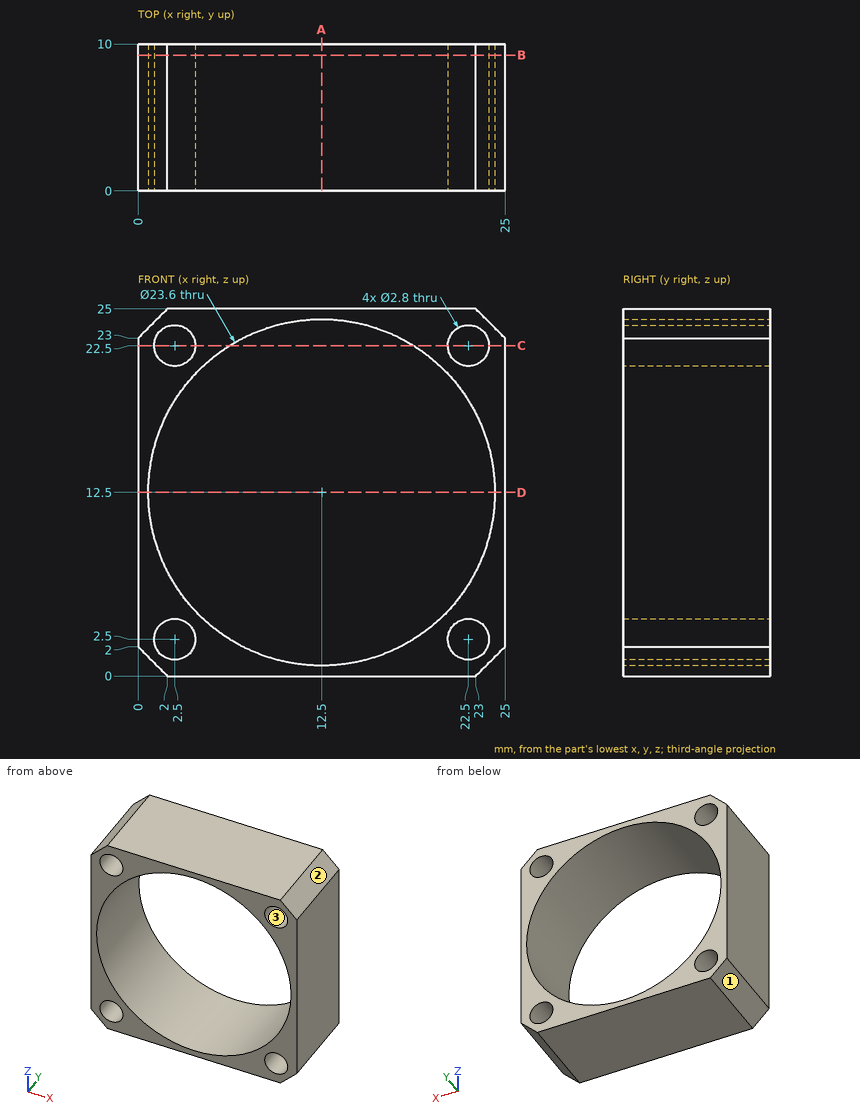
Input: dimensioned drawing with shaded views. Units: mm. Origin: part minimum x, y, z. Round coordinates to 2 decimals unless told otherwise and drop trailing zeros. Loops run counter-clockwise (first coordinate to the right, second up) from the corner with the lowest first, then second, coordinate; pieces in that order, holes last. Notation, with made-up numbers: M 61,-0.5 L 116,-0.5 A24 ccw 116,25.5 Z; hole C -2,3.25 d8. An arc over 180 degrees is marked long. Return JSON: item names as keys, results as strings. Group by question number.
1. Mould query, pull axis Z, two halves, no side actions, for the marked faces 1, 2 and 3. Classes: released by +Z, released by -Z, zero draft, split by the parting line, or undercut.
2. Section query D-D on z = 12.5. Output: boundary loops of the cut face in (x, y).
3. Section query A-A on x = 12.5. Output: boundary loops of the cut face in (y, z), and give its area (3 significant figures).
4. Pin query (flat end, axial travel): pin 1 (2 mm diameter, centred on x = 22.5, z = 2.5, fed in from -Y); pin 2 (6 mm diameter, centred on x = 18, z = 4, fed in from -Y). Return the tip coordinate at first contact, or that it passes through.
5. Material intervals for line 1 along X through (y, z) = (7.5, 2.5); line 2 along X through (y, z) = (1.5, 9); line 3 along Z through (x, y) = (23, 2), sorted ascending. Write a range as from..to.
6. Section query B-B on y = 9.25. Output: boundary loops of the cut face in (x, z).
7. Section query C-C on z = 22.5. Output: boundary loops of the cut face in (x, y), and give its area (3 significant figures).
Checks:
{
 "1": {"face 1": "released by -Z", "face 2": "released by +Z", "face 3": "undercut"},
 "2": {"outline": "M 0,0 L 0.7,0 L 0.7,10 L 0,10 Z; M 24.3,0 L 25,0 L 25,10 L 24.3,10 Z"},
 "3": {"outline": "M 0,0 L 10,0 L 10,0.7 L 0,0.7 Z; M 0,24.3 L 10,24.3 L 10,25 L 0,25 Z", "area": "14.0 mm²"},
 "4": {"pin 1": "passes through", "pin 2": "stops at y = 0"},
 "5": {"line 1": "x = 0..1.1, 3.9..6.24, 18.76..21.1, 23.9..25", "line 2": "x = 0..1.23, 23.77..25", "line 3": "z = 0..1.19, 3.81..7.12, 17.88..21.19, 23.81..25"},
 "6": {"outline": "M 0,2 L 2,0 L 23,0 L 25,2 L 25,23 L 23,25 L 2,25 L 0,23 Z; hole C 12.5,12.5 d23.6; hole C 2.5,2.5 d2.8; hole C 2.5,22.5 d2.8; hole C 22.5,2.5 d2.8; hole C 22.5,22.5 d2.8"},
 "7": {"outline": "M 0,0 L 1.1,0 L 1.1,10 L 0,10 Z; M 3.9,0 L 6.24,0 L 6.24,10 L 3.9,10 Z; M 18.76,0 L 21.1,0 L 21.1,10 L 18.76,10 Z; M 23.9,0 L 25,0 L 25,10 L 23.9,10 Z", "area": "68.7 mm²"}
}
